from build123d import *

# Parameters (mm, degrees)
SKETCH_1_W          = 76.2
SKETCH_1_H          = 30
EXTRUDE_1_DEPTH     = 3
SKETCH_2_W          = 19.6215
SKETCH_2_H          = 3
CUT_EXTRUDE_1_DEPTH = 3
SKETCH_3_W          = 3
SKETCH_3_H          = 9.055
CUT_EXTRUDE_2_DEPTH = 3
EXTRUDE_2_DEPTH     = 3
SKETCH_6_W          = 30.7975
SKETCH_6_H          = 3
EXTRUDE_3_DEPTH     = 3
SKETCH_7_W          = 16.002
SKETCH_7_H          = 12.7
CUT_EXTRUDE_3_DEPTH = 3
SKETCH_8_R          = 4.85
CUT_EXTRUDE_4_DEPTH = 3
FILLET_1_R          = 2.54
SKETCH_9_W          = 3
SKETCH_9_H          = 8.89
CUT_EXTRUDE_5_DEPTH = 3


with BuildPart() as part:
    # 스케치1 → 보스-돌출1 (new body)
    with BuildSketch(Plane.XY):
        Rectangle(SKETCH_1_W, SKETCH_1_H)
    extrude(amount=EXTRUDE_1_DEPTH)

    # 스케치2 → 컷-돌출1 (cut)
    with BuildSketch(Plane.XY.offset(3)):
        with Locations((-28.28925, -13.5)):
            Rectangle(SKETCH_2_W, SKETCH_2_H)
        with Locations((28.28925, -13.5)):
            Rectangle(SKETCH_2_W, SKETCH_2_H)
    extrude(amount=-CUT_EXTRUDE_1_DEPTH, mode=Mode.SUBTRACT)

    # 스케치3 → 컷-돌출2 (cut)
    with BuildSketch(Plane.XY.offset(3)):
        with Locations((-36.6, 10.4725)):
            Rectangle(SKETCH_3_W, SKETCH_3_H)
        with Locations((-36.6, -7.4725)):
            Rectangle(SKETCH_3_W, SKETCH_3_H)
        with Locations((36.6, 10.4725)):
            Rectangle(SKETCH_3_W, SKETCH_3_H)
        with Locations((36.6, -7.4725)):
            Rectangle(SKETCH_3_W, SKETCH_3_H)
    extrude(amount=-CUT_EXTRUDE_2_DEPTH, mode=Mode.SUBTRACT)

    # 스케치5 → 보스-돌출2 (add)
    with BuildSketch(Plane.XY.offset(3)):
        Polygon((44.45, -12), (68.760909196, -12), (44.45, 15), (38.1, 15), (38.1, -12), align=None)
    extrude(amount=-EXTRUDE_2_DEPTH)

    # 스케치6 → 보스-돌출3 (add)
    with BuildSketch(Plane.XY.offset(3)):
        with Locations((0, 16.5)):
            Rectangle(SKETCH_6_W, SKETCH_6_H)
    extrude(amount=-EXTRUDE_3_DEPTH)

    # 스케치7 → 컷-돌출3 (cut)
    with BuildSketch(Plane(origin=(0, 0, 0), x_dir=(-1, 0, 0), z_dir=(0, 0, -1))):
        with Locations((-24.099, -2.65)):
            Rectangle(SKETCH_7_W, SKETCH_7_H)
    extrude(amount=-CUT_EXTRUDE_3_DEPTH, mode=Mode.SUBTRACT)

    # 스케치8 → 컷-돌출4 (cut)
    with BuildSketch(Plane(origin=(0, 0, 0), x_dir=(-1, 0, 0), z_dir=(0, 0, -1))):
        with Locations((-49.53, -5.42)):
            Circle(SKETCH_8_R)
    extrude(amount=-CUT_EXTRUDE_4_DEPTH, mode=Mode.SUBTRACT)

    # 필렛1
    fillet_1_edges = [part.edges().sort_by_distance(p)[0] for p in [
        (44.45, 15, 1.5),
    ]]
    fillet(fillet_1_edges, radius=FILLET_1_R)

    # 스케치9 → 컷-돌출5 (cut)
    with BuildSketch(Plane(origin=(0, 0, 0), x_dir=(-1, 0, 0), z_dir=(0, 0, -1))):
        with Locations((13.1, -4.4802)):
            Rectangle(SKETCH_9_W, SKETCH_9_H)
    extrude(amount=-CUT_EXTRUDE_5_DEPTH, mode=Mode.SUBTRACT)


solid = part.part
For this review, take the finished solid that the model builds, in its own axes (mm). A direction names the side the tool comes from. Round coordinates to 2 decimals unless told otherwise and drop trailing zeros. Loops run counter-clockwise (first coordinate to the right, second up) from the corner with the lowest first, then second, coordinate; pieces in that order, holes last. Notation, with made-up numbers: (12.5, 9) - (44.5, 9) arc R15 cw to (44.5, 23) - close; hole circle Ø3 at (58, -14.75). An arc over 180 degrees is marked (long way). One line per question, with ' | ' between items.
Q1. Tool access review of faces 1 (the flat face through (38.1, -7, 2)), 2 (the flat face through (-37, 5.945, 2)), 3 (the flat face through (24, -9, 1)): name each direction out of +Z, -Z, +X, -X, +Y, -Y from which nothing blocks a thin tool from reaching the whole face with its end or side.
Taken from the geometry:
face 1: +Z, -Z, -Y | face 2: +Z, -Z, -X, +Y | face 3: +Z, -Z
Q2. The part is to be moulded in two halves that separate along X. For faces 4 (the flat face through (-38.1, 1, 1)), 5 (the flat face through (35.1, 10, 2)), 6 (the flat face through (3, 2, 0)), say which applies: released by +X, released by -X, zero draft, split by the parting line, or undercut.
Taken from the geometry:
face 4: released by -X | face 5: undercut | face 6: zero draft
Q3. Take a section at B-B (x = 22). Give the boundary of the cut face in (y, z).
Taken from the geometry:
outline: (-12, 0) - (-9, 0) - (-9, 3) - (-12, 3) - close; (3.7, 0) - (15, 0) - (15, 3) - (3.7, 3) - close
Q4. For line 1 along X through (y, z) = (-9.5, 2.5); line 2 along X through (y, z) = (-2, 0.4); line 3 along X through (y, z) = (-6.5, 0.4), list the stretches that pass through material, from the lowest coordinate up. Write a range as [from, to].
Taken from the geometry:
line 1: x = [-35.1, 35.1], [38.1, 46.91], [52.15, 66.51] | line 2: x = [-38.1, -14.6], [-11.6, 16.1], [32.1, 46.09], [52.97, 59.76] | line 3: x = [-35.1, -14.6], [-11.6, 16.1], [32.1, 35.1], [38.1, 44.8], [54.26, 63.81]
Q5. For pin 1 (0.9 mm diameter, centred on y = -1.5, z = 1, fed in from +X); pin 2 (6 mm diameter, centred on x = -12, y = 11, fed in from -Z); pin 3 (1.5 mm diameter, centred on x = 37, z = 1, fed in from +Y) (3 decimals); pin 4 (0.9 mm diameter, centred on y = -14, z = 1, fed in from -X), all flat-tipped, find the tip position at first contact; note any pin that passes through.
Taken from the geometry:
pin 1: stops at x = 59.71 | pin 2: stops at z = 0 | pin 3: stops at y = 5.945 | pin 4: stops at x = -18.48
Q6. Take a section at D-D (y = 12.5). Give the boundary of the cut face in (x, z), and give its area (3 significant figures).
Taken from the geometry:
outline: (-35.1, 0) - (35.1, 0) - (35.1, 3) - (-35.1, 3) - close; (38.1, 0) - (46.7, 0) - (46.7, 3) - (38.1, 3) - close | area: 236 mm²
Q7. Take a section at C-C (y = -8). Give the boundary of the cut face in (x, z), and give its area (3 significant figures).
Taken from the geometry:
outline: (-35.1, 0) - (-14.6, 0) - (-14.6, 3) - (-35.1, 3) - close; (-11.6, 0) - (16.1, 0) - (16.1, 3) - (-11.6, 3) - close; (32.1, 0) - (35.1, 0) - (35.1, 3) - (32.1, 3) - close; (38.1, 0) - (45.42, 0) - (45.42, 3) - (38.1, 3) - close; (53.64, 0) - (65.16, 0) - (65.16, 3) - (53.64, 3) - close | area: 210 mm²
Q8. Take a section at A-A (z = 0.5). State how many separate pieces and enclosed holes the cut face has, and give its area (3 significant figures).
Taken from the geometry:
separate pieces: 1 | enclosed holes: 3 | area: 2,350 mm²
